Autodesk Inventor part; units mm, degrees
ref_plane "Work Plane2" through (0, 0, 4) normal (0, 0, 1) x (1, 0, 0)
ref_plane "Work Plane8" through (0, 0, 0) normal (0.9238795, 0.3826834, 0) x (0, 0, 1)
ref_plane "Work Plane9" through (0, 0, 0) normal (1, 0, 0) x (0, 1, 0)
sketch "Sketch1" plane through (0, 0, 0) normal (0, 0, 1) x (1, 0, 0)
  circle A0 centre (0, 0) radius 10
  dimension "d0" = 20
extrude "Extrusion1" add sketch "Sketch1" along normal blind 8
ref_plane "Work Plane2" through (0, 0, 4) normal (0, 0, 1) x (1, 0, 0)
sketch "Sketch2" plane through (0, 0, 0) normal (0, 0, -1) x (-1, 0, 0)
  circle A0 centre (0, 0) radius 10
  circle A1 centre (0, 0) radius 8
  dimension "d3" = 16
surface extrude "Pitch Diameter" sketch "Sketch2" against normal through all shown no curves A1
ref_plane "Work Plane8" through (0, 0, 0) normal (0.9238795, 0.3826834, 0) x (0, 0, 1)
ref_plane "Work Plane9" through (0, 0, 0) normal (1, 0, 0) x (0, 1, 0)
spur gear teeth "Spur Gear" teeth 8 pitch diameter 16 tip diameter 20 root diameter 11 face width 8 start plane through (0, 0, 0) normal (0, 0, -1) x (-1, 0, 0)
sketch "Sketch3" plane through (0, 0, 8) normal (0, 0, 1) x (1, 0, 0)
  circle A0 centre (0, 0) radius 3.5
  dimension "d52" = 7
extrude "Extrusion2" cut sketch "Sketch3" against normal through all
equation "\"d0\" = da_da"
equation "\"d1\" = da_b"
equation "\"d3\" = da_d"
equation "\"d16\" = da_aw"
equation "\"d43\" = da_aw"
equation "\"d46\" = da_aw"
properties part number "Spur Gear1" material "Steel"
Here's how the part is built. I have some questions about the finished solid (model axes, mm). A direction names the side the tool comes from. Coordinates: 2 decimals unless noted, no trailing zeros. Loops run counter-clockwise (first coordinate to the right, second up) from the corner with the lowest first, then second, coordinate; pieces in that order, holes last. Notation, with made-up numbers: (51, 50) - (104, 50) arc R22 ccw to (104, 72) - close; hole circle Ø3 at (78, -7.5). An arc over 180 degrees is marked (long way). Return JSON: item names as keys, results as strings. Group by question number.
Item 1: If we section it at A-A on y = 0: Write out the boundary of the cut face in (x, z).
Item 2: We'd pull the mould along X, two halves only. Please class faces 1 (the face through (2.098, 5.084, 3.944)), 2 (the face through (0, -4, 0)), 3 (the face through (-1.585, -7.68, 3.944)), 4 (the face through (6.55, 4.31, 3.94)): +X half, -X half, draft (parallel to the pull), parting line (faces both ways), or undercut.
Item 3: On a 3-axis mill with a long thin cutter (end or side, diameter ignored), from which of +Z, -Z, +X, -X, +Y, -Y can I reach the whole of each face in a straight line? I mean faces 5 (the face through (1.585, 7.68, 3.944)), 6 (the face through (-6.511, 4.257, 3.944)), 7 (the face through (4.31, -6.55, 3.94)), 8 (the face through (6.511, -4.257, 3.944)), 9 (the face through (4.257, 6.511, 3.944)). Say none if no direction works.
Item 4: If we section it at D-D on x = -7: Write out the boundary of the cut face in (y, z).
Item 5: I need wall thicknesses on line 1 (Y direction, x = 0, z = 2.25); line 2 (X direction, y = -7.25, z = 5); line 3 (X direction, y = 2.25, z = 2.5). Which ranges of each line are inside material? Lowest first, please. Write a range as from..to.
Item 6: Will these pins go through, and if not, where does the flat tip stop? P1, Ø1, axis at x = -2.5, y = -7, coming from the -Z side; P2, Ø1, axis at x = 1, z = 5.5, coming from the +Y side; P3, Ø1.5, axis at y = -5, z = 1, coming from the +X side.
Calculated:
{
 "1": {"outline": "(-10, 0) - (-3.5, 0) - (-3.5, 8) - (-10, 8) - close; (3.5, 0) - (10, 0) - (10, 8) - (3.5, 8) - close"},
 "2": {"face 1": "undercut", "face 2": "draft", "face 3": "undercut", "face 4": "+X half"},
 "3": {"face 5": "+Z, -Z", "face 6": "+Z, -Z, -X", "face 7": "+Z, -Z, -Y", "face 8": "+Z, -Z, +X", "face 9": "+Z, -Z, +Y"},
 "4": {"outline": "(-7.14, 0) - (-4.95, 0) - (-4.95, 8) - (-7.14, 8) - close; (-1.65, 0) - (1.65, 0) - (1.65, 8) - (-1.65, 8) - close; (4.95, 0) - (7.14, 0) - (7.14, 8) - (4.95, 8) - close"},
 "5": {"line 1": "y = -10..-3.5, 3.5..10", "line 2": "x = -6.89..-5.37, -1.63..1.63, 5.37..6.89", "line 3": "x = -5.02..-2.68, 2.68..5.02"},
 "6": {"P1": "passes through", "P2": "stops at y = 9.99", "P3": "stops at x = 7.45"}
}
